```python
from build123d import *

# Parameters (mm, degrees)
SKETCH_1_W          = 71
SKETCH_1_H          = 32
SKETCH_1_R          = 1.45
EXTRUDE_1_DEPTH     = 5
SKETCH_2_R          = 1.6
CUT_EXTRUDE_1_DEPTH = 5
FILLET_1_R          = 2


with BuildPart() as part:
    # 草图1 → 凸台-拉伸1 (new body)
    with BuildSketch(Plane(origin=(0, 0, 0), x_dir=(1, 0, 0), z_dir=(0, 1, 0))):
        Rectangle(SKETCH_1_W, SKETCH_1_H)
        with Locations(Location((14.5, -10, 0), (0, 0, 270))):
            Circle(SKETCH_1_R, mode=Mode.SUBTRACT)
    extrude(amount=EXTRUDE_1_DEPTH)

    # 草图2 → 切除-拉伸1 (cut)
    with BuildSketch(Plane(origin=(0, 5, 0), x_dir=(1, 0, 0), z_dir=(0, 1, 0))):
        with Locations(Location((-31.5, 12, 0), (0, 0, 270))):
            Circle(SKETCH_2_R)
        with Locations(Location((-31.5, -12, 0), (0, 0, 270))):
            Circle(SKETCH_2_R)
        with Locations(Location((31.5, 12, 0), (0, 0, 270))):
            Circle(SKETCH_2_R)
    extrude(amount=-CUT_EXTRUDE_1_DEPTH, mode=Mode.SUBTRACT)

    # 圆角1
    fillet_1_edges = [part.edges().sort_by_distance(p)[0] for p in [
        (35.5, 2.5, 16),
        (-35.5, 2.5, 16),
        (-35.5, 2.5, -16),
        (35.5, 2.5, -16),
    ]]
    fillet(fillet_1_edges, radius=FILLET_1_R)


solid = part.part
```
For this review, take the finished solid that the model builds, in its own axes (mm). Round coordinates to 2 decimals unless told otherwise and drop trailing zeros. Write each loop counter-clockwise with the first axis right and the second up, starting at its lowest first coordinate (ties: lowest second). Pieces come first, ordered by that corner, then holes. Notation, with made-up numbers: M -31,-22.75 L -4,-22.75 A33 ccw -4,14.25 Z; hole C -31.75,-0.5 d7. An arc over 180 degrees is marked long. One line per item, written item: value. Start each with the question number.
(1) We need section B-B (z = -12). Give the boundary of the cut face in (x, y).
(2) We need section C-C (x = 14.5). Give the boundary of the cut face in (y, z).
(3) The part is to be moulded in two halves that separate along X. For faces 1 (the flat face through (0, 2, 16)), 2 (the cylindrical face through (14.56, 2.46, 8.55)), 3 (the cylindrical face through (34.9, 2.54, -15.43)), 4 (the cylindrical face through (-31.43, 2.54, 10.4)), say which applies: released by +X, released by -X, zero draft, split by the parting line, or undercut.
(4) Wall thickness on line 1 (X direction, y = 1.25, z = -12); line 2 (X direction, y = 1.45, z = 10); line 3 (X direction, y = 3.9, z = -11): over which ranges is each line inside the solid? List them lowest first.
(5) We need section A-A (y = 1). Give the boundary of the cut face in (x, z).
(6) We need section D-D (x = 31.5). Give the boundary of the cut face in (y, z), and give its area (3 significant figures).
Result:
1. outline: M -35.5,0 L -33.1,0 L -33.1,5 L -35.5,5 Z; M -29.9,0 L 29.9,0 L 29.9,5 L -29.9,5 Z; M 33.1,0 L 35.5,0 L 35.5,5 L 33.1,5 Z
2. outline: M 0,-16 L 5,-16 L 5,8.55 L 0,8.55 Z; M 0,11.45 L 5,11.45 L 5,16 L 0,16 Z
3. face 1: zero draft
3. face 2: undercut
3. face 3: released by +X
3. face 4: undercut
4. line 1: -35.5 to -33.1, -29.9 to 29.9, 33.1 to 35.5
4. line 2: -35.5 to 13.05, 15.95 to 35.5
4. line 3: -35.5 to -32.75, -30.25 to 30.25, 32.75 to 35.5
5. outline: M -35.5,-14 A2 ccw -33.5,-16 L 33.5,-16 A2 ccw 35.5,-14 L 35.5,14 A2 ccw 33.5,16 L -33.5,16 A2 ccw -35.5,14 Z; hole C -31.5,-12 d3.2; hole C -31.5,12 d3.2; hole C 14.5,10 d2.9; hole C 31.5,-12 d3.2
6. outline: M 0,-16 L 5,-16 L 5,-13.6 L 0,-13.6 Z; M 0,-10.4 L 5,-10.4 L 5,16 L 0,16 Z
6. area: 144 mm²
